Verification items for this drawing (mm, ordinates from the low corner). A direction names the side the tool comes from. Coordinates: 2 decimals unless noted, no trailing zeros. Loops run counter-clockwise (first coordinate to the right, second up) from the corner with the lowest first, then second, coordinate; pieces in that order, holes last. Notation, with made-up numbers: (36.25, -18) - (79.25, -18) arc R15 ccw to (79.25, -2) - close; hole circle Ø1 at (32.5, -4). An arc over 180 degrees is marked (long way). Write each question's results on one line, items separated by ' | '. Start each with the question number.
(1) Mould release check, pull along Y, two halves, no side actions. Record for the marked faces 5, 6 and 7: pulls with the +Y half, pulls with the -Y half, needs draft (parallel to the pull), parting line crosses it, or undercut.
(2) Access from +Z, -Z, +X, -X, +Y, -Y to the whole of each face (thin tool, end or side, straight path). Record for the marked faces 1, 2, 3 and 4.
(3) Go/stop test with flat-tipped pins: pin 1 Ø2 at (x, y) = (18.5, 58.5) entering from +Z; pin 2 Ø4.5 at (x, z) = (17.5, 43) entering from -Y; pin 3 Ø7 at (y, z) = (48.5, 29) entering from +X; pin 4 Ø7 at (y, z) = (52, 25.5) entering from -X. Record where each tip stops, or that it passes through.
(4) Sectioned sample at C-C (y = 54.15). Enter the section's corners in (x, z).
(5) Sectioned sample at A-A (x = 17.5). Enter the section's corners in (y, z), plus the area to 3 significant figures.
(6) Material ranges on probe 1 along X at (y, z) = (4.5, 43); probe 2 along Z at (x, y) = (33, 61); probe 3 along X at (y, z) = (58.5, 7), recorded low to high.
(7) Sectioned sample at D-D (x = 9). Enter the section's corners in (y, z), plus the area to 3 significant figures.
(8) Sectioned sample at B-B (z = 43). Enter the section's corners in (x, y), plus the area to 4 significant figures.
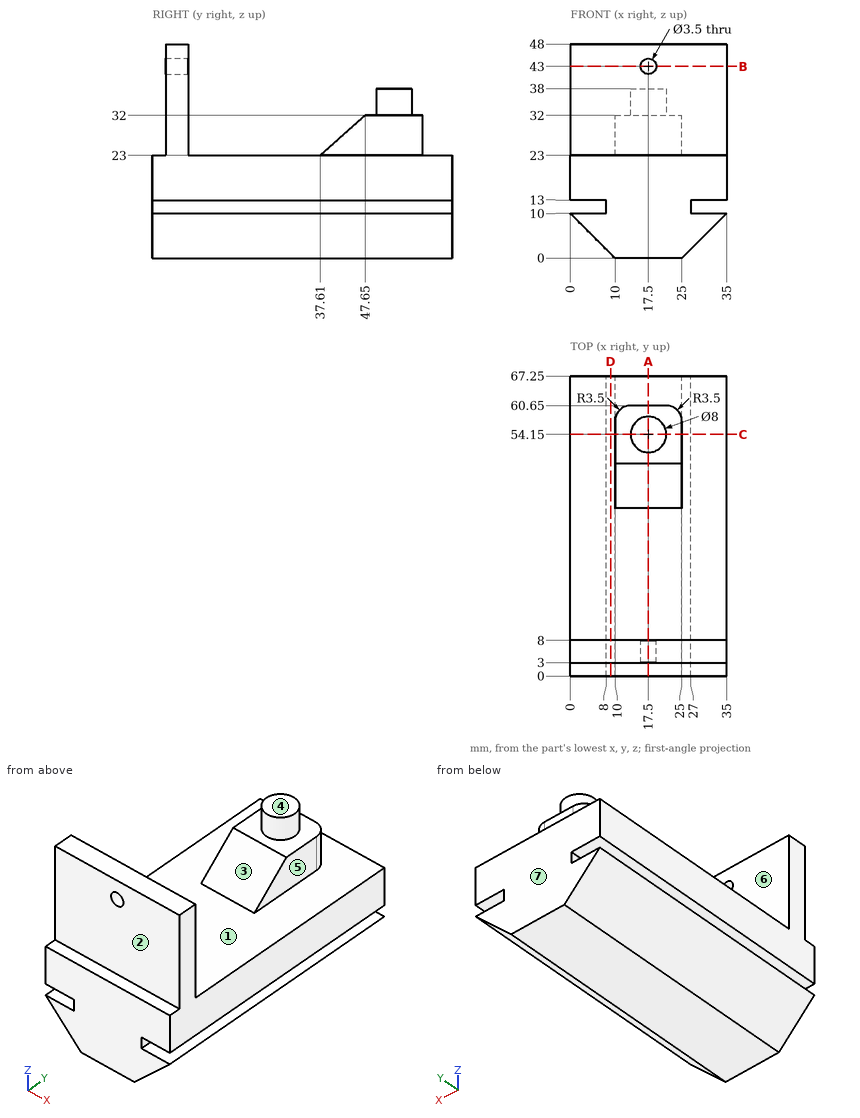
Outcome:
1) face 5: needs draft | face 6: undercut | face 7: pulls with the +Y half
2) face 1: +Z | face 2: +Z, +X, -X, -Y | face 3: +Z, +X, -X | face 4: +Z, +X, -X, +Y
3) pin 1: stops at z = 38 | pin 2: stops at y = 3 | pin 3: stops at x = 25 | pin 4: stops at x = 0
4) outline: (0, 10) - (10, 0) - (25, 0) - (35, 10) - (27, 10) - (27, 13) - (35, 13) - (35, 23) - (25, 23) - (25, 32) - (21.5, 32) - (21.5, 38) - (13.5, 38) - (13.5, 32) - (10, 32) - (10, 23) - (0, 23) - (0, 13) - (8, 13) - (8, 10) - close
5) outline: (0, 0) - (67.25, 0) - (67.25, 23) - (60.65, 23) - (60.65, 32) - (58.15, 32) - (58.15, 38) - (50.15, 38) - (50.15, 32) - (47.65, 32) - (37.61, 23) - (8, 23) - (8, 41.25) - (3, 41.25) - (3, 23) - (0, 23) - close; (3, 44.75) - (8, 44.75) - (8, 48) - (3, 48) - close | area: 1,860 mm2
6) probe 1: x = 0 to 15.75, 19.25 to 35 | probe 2: z = 8 to 10, 13 to 23 | probe 3: x = 3 to 32
7) outline: (0, 1) - (67.25, 1) - (67.25, 23) - (8, 23) - (8, 48) - (3, 48) - (3, 23) - (0, 23) - close | area: 1,600 mm2
8) outline: (0, 3) - (15.75, 3) - (15.75, 8) - (0, 8) - close; (19.25, 3) - (35, 3) - (35, 8) - (19.25, 8) - close | area: 157.5 mm2
